Autodesk Fusion 360 part; units mm, degrees
sketch "Skizze1" plane through (0, 0, 0) normal (0, 0, 1) x (1, 0, 0)
  line L0 (0, 0) -> (230, 0)
  line L1 (230, 0) -> (230, 20)
  line L2 (230, 20) -> (205, 20)
  line L3 (230, 30) -> (205, 30)
  line L4 (230, 30) -> (230, 50)
  line L5 (230, 50) -> (200, 50)
  line L6 (170, 50) -> (175, 40)
  line L7 (175, 40) -> (195, 40)
  line L8 (200, 50) -> (195, 40)
  line L9 (55, 40) -> (35, 40)
  line L10 (55, 40) -> (60, 50)
  line L11 (35, 40) -> (30, 50)
  line L12 (30, 50) -> (0, 50)
  line L13 (0, 50) -> (0, 30)
  line L14 (0, 30) -> (25, 30)
  line L15 (0, 0) -> (0, 20)
  line L16 (0, 20) -> (25, 20)
  arc A0 (25, 20) -> (25, 30) centre (25, 25) ccw
  arc A1 (205, 30) -> (205, 20) centre (205, 25) ccw
  line L17 (115, 40) -> (79, 40)
  line L18 (115, 40) -> (151, 40)
  line L19 (79, 40) -> (79, 15)
  line L20 (79, 15) -> (151, 15)
  line L21 (151, 15) -> (151, 40)
  circle A2 centre (100, 45) radius 1.6
  circle A3 centre (130, 45) radius 1.6
  line L22 (60, 50) -> (170, 50)
  dimension "d1" = 230
  dimension "d2" = 20
  dimension "d3" = 25
  dimension "d6" = 10
  dimension "d7" = 25
  dimension "d8" = 20
  dimension "d9" = 30
  dimension "d11" = 30
  dimension "d14" = 20
  dimension "d15" = 110
  dimension "d18" = 20
  dimension "d20" = 30
  dimension "d21" = 20
  dimension "d22" = 25
  dimension "d23" = 20
  dimension "d24" = 25
  dimension "d27" = 36
  dimension "d28" = 36
  dimension "d29" = 25
  dimension "d30" = 72
  dimension "d33" = 3.2
extrude "Extrusion1" add sketch "Skizze1" along normal blind 10
sketch "Skizze2" plane through (230, 0, 0) normal (1, 0, 0) x (0, 1, 0)
  line L0 (0, 0) -> (20, 0)
  line L1 (20, 0) -> (20, 10)
  line L2 (20, 10) -> (0, 10)
  line L3 (0, 10) -> (0, 0)
  line L4 (0, 10) -> (20, 0)
  line L5 (20, 10) -> (0, 0)
  line L6 (49.9281, 0) -> (49.9281, 10)
  circle A0 centre (10, 5) radius 1.2
  dimension "d36" = 2.4
sketch "Skizze3" plane through (230, 0, 0) normal (1, 0, 0) x (0, 1, 0)
  line L0 (30, 0) -> (50, 0)
  line L1 (50, 0) -> (50, 10)
  line L2 (50, 10) -> (30, 10)
  line L3 (30, 10) -> (30, 0)
  line L4 (30, 10) -> (50, 0)
  line L5 (50, 10) -> (30, 0)
  circle A0 centre (40, 5) radius 1.2
  dimension "d37" = 2.4
sketch "Skizze4" plane through (0, 0, 0) normal (-1, 0, 0) x (0, -1, 0)
  line L0 (-50, 0) -> (-30, 0)
  line L1 (-30, 0) -> (-30, 10)
  line L2 (-30, 10) -> (-50, 10)
  line L3 (-50, 10) -> (-50, 0)
  line L4 (-50, 10) -> (-30, 0)
  line L5 (-30, 10) -> (-50, 0)
  line L6 (0, 0) -> (0, 10)
  circle A0 centre (-40, 5) radius 1
  dimension "d38" = 2
sketch "Skizze5" plane through (0, 0, 0) normal (-1, 0, 0) x (0, -1, 0)
  line L0 (-20, 0) -> (0, 0)
  line L1 (0, 0) -> (0, 10)
  line L2 (0, 10) -> (-20, 10)
  line L3 (-20, 10) -> (-20, 0)
  line L4 (-20, 10) -> (0, 0)
  line L5 (0, 10) -> (-20, 0)
  circle A0 centre (-10, 5) radius 1
  dimension "d39" = 2
hole "Bohrung1" at (230, 10, 5) direction (-1, 0, 0) diameter 2.4 depth 20 tip angle 118
hole "Bohrung2" at (230, 40, 5) direction (-1, 0, 0) diameter 2.4 depth 20 tip angle 118
hole "Bohrung3" at (0, 10, 5) direction (1, 0, 0) diameter 2.4 depth 20 tip angle 118
hole "Bohrung4" at (0, 40, 5) direction (1, 0, 0) diameter 2.4 depth 20 tip angle 118
equation "d36 = Montagelochdurchmesser"
equation "d37 = Montagelochdurchmesser"
equation "d41 = Montagelochdurchmesser"
equation "d44 = Montagelochdurchmesser"
equation "d47 = Montagelochdurchmesser"
equation "d50 = Montagelochdurchmesser"
equation "Montagelochdurchmesser = 2.4 mm"
Can you work these out from the model? Positions are in its coordinate system, mm. A direction names the side the tool comes from. Give positions to 0.01 mm unless a question says otherwise; leave off trailing zeros. Order: outer loops, then holes, each group sorted by start corner. A loop starts at its lowest first (then second) coordinate and runs counter-clockwise, first axis right, second up. Notation, with made-up numbers: M 87.25,33.5 L 144.25,33.5 A19 ccw 144.25,40.5 Z; hole C 64,81 d8. An arc over 180 degrees is marked long. Use a Markdown table: item, result. Add a question column.
Item 1: Suppose I cut it at A-A (y = 25). List the corners of the cut face in (x, z) for me, then the cut area to 3 significant figures.
Item 2: Will these pins go through, and if not, where does the flat tip stop? pin 1 (5 mm diameter, centred on y = 26.5, z = 7, fed in from -X); pin 2 (1.4 mm diameter, centred on y = 10, z = 5, fed in from -X); pin 3 (1 mm diameter, centred on y = 23, z = 1.5, fed in from -X); pin 4 (8 mm diameter, centred on x = 113.5, y = 35.5, fed in from -Z).
Item 3: Suppose I cut it at B-B (z = 8). List the corners of the cut face in (x, y) for me, then the cut area to 3 significant figures.
Item 4: We'd pull the mould along Y, two halves only. Please class faces 1 (the flat face through (79, 28, 5)), 2 (the flat face through (113, 0, 5)), 3 (the flat face through (230, 38, 5)), 4 (the flat face through (32.535, 44.93, 4.93)): +Y half, -Y half, draft (parallel to the pull), parting line (faces both ways), or undercut.
Item 5: If I drill on L1, parallel to Y at x = 130, z = 3.75; L2, parallel to Y at x = 225.5, z = 5; L3, parallel to Y at x = 128, z = 5.75, over which ranges is the centre line in solid material (lowest first)? Write a range as [from, to].
Item 6: For faces 5 (the flat face through (45, 40, 5)), 6 (the flat face through (116, 40, 5)), 7 (the flat face through (218, 20, 5)), 8 (the cylindrical face through (30, 25, 5)), which set-ups out of +Z, -Z, +X, -X, +Y, -Y let a thin tool reach every point of the face, with its end or its side?
Answer sheet:
| question | item | result |
|---|---|---|
| 1 | outline | M 30,0 L 79,0 L 79,10 L 30,10 Z; M 151,0 L 200,0 L 200,10 L 151,10 Z |
| 1 | area | 980 mm² |
| 2 | pin 1 | stops at x = 28 |
| 2 | pin 2 | stops at x = 20.3 |
| 2 | pin 3 | stops at x = 29.33 |
| 2 | pin 4 | passes through |
| 3 | outline | M 0,0 L 230,0 L 230,20 L 205,20 A5 cw 205,30 L 230,30 L 230,50 L 200,50 L 195,40 L 175,40 L 170,50 L 60,50 L 55,40 L 35,40 L 30,50 L 0,50 L 0,30 L 25,30 A5 cw 25,20 L 0,20 Z; hole M 79,15 L 151,15 L 151,40 L 79,40 Z; hole C 100,45 d3.2; hole C 130,45 d3.2 |
| 3 | area | 8,610 mm² |
| 4 | face 1 | undercut |
| 4 | face 2 | -Y half |
| 4 | face 3 | draft |
| 4 | face 4 | +Y half |
| 5 | L1 | y = [0, 15], [40, 43.4], [46.6, 50] |
| 5 | L2 | y = [0, 8.8], [11.2, 20], [30, 38.8], [41.2, 50] |
| 5 | L3 | y = [0, 15], [40, 50] |
| 6 | face 5 | +Z, -Z, +Y |
| 6 | face 6 | +Z, -Z |
| 6 | face 7 | +Z, -Z, +X |
| 6 | face 8 | +Z, -Z, -X |
